Build history of the part. All positions in model axes, mm. A direction names the side the tool comes from. Give positions to 0.01 mm unless a question says otherwise; leave off trailing zeros. Order: outer loops, then holes, each group sorted by start corner. A loop starts at its lowest first (then second) coordinate and runs counter-clockwise, first axis right, second up. Notation, with made-up numbers: (82.5, 66.5) -> (97.5, 66.5) arc R14 cw to (97.5, 72.5) -> close; hole circle Ø2 at (13.5, 84.25). An arc over 180 degrees is marked (long way). One line per item, written item: value. Start each with the question number.
(1) Saw through at C-C on x = -17. Give the cut face in (y, z).
(2) Probe line 1 (X direction, y = 17.5, z = 1.95); line 2 (Y direction, x = 0, z = 2.95); line 3 (X direction, y = 32, z = 1.05). List the from-to ranges inside material, lowest first.
(3) Saw through at D-D on x = -10. Give the cut face in (y, z).
(4) Pin check, flat tips, straight feed: pin 1 (6 mm diameter, centred on x = -2.5, y = -27, fed in from -Z); pin 2 (1.8 mm diameter, centred on x = -17.64, y = 17.64, fed in from +Z); pin 3 (2 mm diameter, centred on x = -19, z = 2.5, fed in from +Y); pin 4 (1.2 mm diameter, centred on y = 34, z = 2.5, fed in from -X). Stop position of each tip, or through.
(5) Saw through at A-A on y = 0. Give the cut face in (x, z), plus the area to 3 significant figures.
(6) Which spindle directions (+Z, -Z, +X, -X, +Y, -Y) get a long thin tool onto all of the face, cutting with end or side? Do faces 4 (the flat face through (-22, 32.3, 2)), 5 (the cylindrical face through (-2.38, 10.74, 1.97)), 6 (the flat face through (-23, -32.3, 2)). Say none if no direction does.
(7) Saw through at B-B on x = 0. Give the cut face in (y, z).
(8) Two-plate mould, pull along Y, no slides. Class faces 1 (the cylindrical face through (16.53, 16.63, 1.97)), 2 (the flat face through (8, -37.3, 2)), 3 (the flat face through (-30, 0, 2)): +Y half, -Y half, draft (parallel to the pull), parting line (faces both ways), or undercut.
Autodesk Inventor part; units mm, degrees
ref_plane "YZ Plane" through (0, 0, 0) normal (1, 0, 0) x (0, 1, 0)
ref_plane "XZ Plane" through (0, 0, 0) normal (0, 1, 0) x (-1, 0, 0)
ref_plane "XY Plane" through (0, 0, 0) normal (0, 0, 1) x (1, 0, 0)
sketch "Sketch1" plane through (0, 0, 0) normal (0, 0, 1) x (1, 0, 0)
  circle A0 centre (0, 0) radius 11
  line L0 (-15, 37.3) -> (30, 37.3)
  line L1 (30, 37.3) -> (30, -37.3)
  line L2 (30, -37.3) -> (-15, -37.3)
  line L3 (-15, -37.3) -> (-15, 37.3)
  line L4 (-15, 32.3) -> (-30, 32.3)
  line L5 (-30, 32.3) -> (-30, -32.3)
  line L6 (-30, -32.3) -> (-15, -32.3)
  line L7 (-15, -32.3) -> (-15, 32.3)
  circle A1 centre (-10, 32.3) radius 1.5
  circle A2 centre (3, 32.3) radius 1.5
  circle A3 centre (-10, -32.3) radius 1.5
  circle A4 centre (3, -32.3) radius 1.5
  circle A5 centre (-17.6398, 17.6398) radius 1.5
  line L8 (0, 0) -> (-17.6398, 17.6398) construction
  line L9 (0, 0) -> (-30, 0) construction
  circle A6 centre (-17.6398, -17.6398) radius 1.5
  circle A7 centre (17.6398, -17.6398) radius 1.5
  circle A8 centre (17.6398, 17.6398) radius 1.5
  point P0 (-15, -32.3)
  dimension "d0" = 22
  dimension "d1" = 3
  dimension "d2" = 3
  dimension "d3" = 3
  dimension "d4" = 3
  dimension "d5" = 5
  dimension "d6" = 5
  dimension "d7" = 5
  dimension "d8" = 13
  dimension "d9" = 13
  dimension "d10" = 5
  dimension "d11" = 5
  dimension "d12" = 5
  dimension "d13" = 74.6
  dimension "d14" = 37.3
  dimension "d15" = 60
  dimension "d16" = 15
  dimension "d17" = 5
  dimension "d18" = 5
  dimension "d19" = 30
  dimension "d20" = 3
  dimension "d22" = 45
  dimension "d25" = 360
extrude "Extrusion1" add sketch "Sketch1" along normal blind 4
equation "\"d7\" = d6"
equation "\"d9\" = d8"
equation "\"d11\" = d10"
equation "\"d12\" = d10"
equation "\"d18\" = d17"
properties part number "MotorHolder"
Results below:
1. outline: (-32.3, 0) -> (-19, 0) -> (-19, 4) -> (-32.3, 4) -> close; (-16.28, 0) -> (16.28, 0) -> (16.28, 4) -> (-16.28, 4) -> close; (19, 0) -> (32.3, 0) -> (32.3, 4) -> (19, 4) -> close
2. line 1: x = -30 to -19.13, -16.15 to 16.15, 19.13 to 30
2. line 2: y = -37.3 to -11, 11 to 37.3
2. line 3: x = -30 to -11.47, -8.53 to 1.53, 4.47 to 30
3. outline: (-37.3, 0) -> (-33.8, 0) -> (-33.8, 4) -> (-37.3, 4) -> close; (-30.8, 0) -> (-4.58, 0) -> (-4.58, 4) -> (-30.8, 4) -> close; (4.58, 0) -> (30.8, 0) -> (30.8, 4) -> (4.58, 4) -> close; (33.8, 0) -> (37.3, 0) -> (37.3, 4) -> (33.8, 4) -> close
4. pin 1: stops at z = 0
4. pin 2: passes through
4. pin 3: stops at y = 32.3
4. pin 4: stops at x = -15
5. outline: (-30, 0) -> (-11, 0) -> (-11, 4) -> (-30, 4) -> close; (11, 0) -> (30, 0) -> (30, 4) -> (11, 4) -> close
5. area: 152 mm²
6. face 4: +Z, -Z, -X, +Y
6. face 5: +Z, -Z
6. face 6: +Z, -Z, -X, -Y
7. outline: (-37.3, 0) -> (-11, 0) -> (-11, 4) -> (-37.3, 4) -> close; (11, 0) -> (37.3, 0) -> (37.3, 4) -> (11, 4) -> close
8. face 1: undercut
8. face 2: -Y half
8. face 3: draft
